```python
from build123d import *

# Parameters (mm, degrees)
SKETCH1_W           = 7.62
SKETCH1_H           = 19.05
BOSS_EXTRUDE1_DEPTH = 63.5
SKETCH2_R           = 0.889
CUT_EXTRUDE1_DEPTH  = 6.35
SKETCH3_R           = 3.3782
CUT_EXTRUDE2_DEPTH  = 8.62
SKETCH4_R           = 3.3782
CUT_EXTRUDE3_DEPTH  = 8.62


with BuildPart() as part:
    # Sketch1 → Boss-Extrude1 (new body)
    with BuildSketch(Plane.XY):
        with Locations((3.81, 9.525)):
            Rectangle(SKETCH1_W, SKETCH1_H)
    extrude(amount=-BOSS_EXTRUDE1_DEPTH)

    # Sketch2 → Cut-Extrude1 (cut)
    with BuildSketch(Plane.XY):
        with Locations((4.826, 11.43)):
            Circle(SKETCH2_R)
    extrude(amount=-CUT_EXTRUDE1_DEPTH, mode=Mode.SUBTRACT)

    # Sketch3 → Cut-Extrude2 (cut, through all)
    with BuildSketch(Plane.ZY):
        with Locations((-48.26, 12.7)):
            Circle(SKETCH3_R)
    extrude(amount=-CUT_EXTRUDE2_DEPTH, mode=Mode.SUBTRACT)

    # Sketch4 → Cut-Extrude3 (cut, through all)
    with BuildSketch(Plane.ZY):
        with Locations((-26.67, 12.7)):
            Circle(SKETCH4_R)
    extrude(amount=-CUT_EXTRUDE3_DEPTH, mode=Mode.SUBTRACT)


solid = part.part
```
Geometry: final body of the model. Coordinates: model frame, mm. A direction names the side the tool comes from. Round coordinates to 2 decimals unless told otherwise and drop trailing zeros. Order: outer loops, then holes, each group sorted by start corner. A loop starts at its lowest first (then second) coordinate and runs counter-clockwise, first axis right, second up. Notation, with made-up numbers: (10, -16.5) -> (68, -16.5) arc R33 cw to (68, 13.5) -> close; hole circle Ø6 at (70.5, 53). An arc over 180 degrees is marked (long way). Use one line per item in the form item = value. Start each with the question number.
1. Draft query along X for faces 1 (the face through (3.938, 11.469, -3.131)), 2 (the face through (0, 9, -31)), 3 (the face through (4, 0, -31)). Return one class per face: pulls with the +X half, pulls with the -X half, needs draft (parallel to the pull), parting line crosses it, or undercut.
2. Reachability of faces 4 (the face through (4, 19.05, -31)), 5 (the face through (5, 11, -6.35)) from +Z, -Z, +X, -X, +Y, -Y: full face, straight path, thin tool, end or side. Return the list, or none.
3. Line query: probe 1 along Z at (x, y) = (4.75, 14); probe 2 along Y at (x, z) = (2, -26.67); probe 3 along Z at (x, y) = (6.5, 13.25). Output: solid intervals per line, ascending.
4. Cut plane B-B (z = -26.67). Return the cut outline in (x, y), then the cut area to 3 significant figures.
5. Pin query (flat end, axial travel): pin 1 Ø9 at (y, z) = (12.7, -48.26) entering from -X; pin 2 Ø0.5 at (x, y) = (5, 12) entering from +Z. Return the tip coordinate at first contact, or that it passes through.
6. Cut plane C-C (y = 11.43). Return the cut outline in (x, z) (3 decimals).
7. Cut plane A-A (x = 2). Return the cut outline in (y, z), then the cut area to 3 significant figures.
Solution:
q1.face_1 = undercut
q1.face_2 = pulls with the -X half
q1.face_3 = needs draft
q2.face_4 = +Z, -Z, +X, -X, +Y
q2.face_5 = +Z
q3.probe_1 = -63.5 to -51.38, -45.14 to -29.79, -23.55 to 0
q3.probe_2 = 0 to 9.32, 16.08 to 19.05
q3.probe_3 = -63.5 to -51.59, -44.93 to -30, -23.34 to 0
q4.outline = (0, 0) -> (7.62, 0) -> (7.62, 9.32) -> (0, 9.32) -> close; (0, 16.08) -> (7.62, 16.08) -> (7.62, 19.05) -> (0, 19.05) -> close
q4.area = 93.7 mm^2
q5.pin_1 = 0
q5.pin_2 = -6.35
q6.outline = (0, -63.5) -> (7.62, -63.5) -> (7.62, -51.39) -> (0, -51.39) -> close; (0, -45.13) -> (7.62, -45.13) -> (7.62, -29.8) -> (0, -29.8) -> close; (0, -23.54) -> (7.62, -23.54) -> (7.62, 0) -> (5.715, 0) -> (5.715, -6.35) -> (3.937, -6.35) -> (3.937, 0) -> (0, 0) -> close
q7.outline = (0, -63.5) -> (19.05, -63.5) -> (19.05, 0) -> (0, 0) -> close; hole circle Ø6.76 at (12.7, -48.26); hole circle Ø6.76 at (12.7, -26.67)
q7.area = 1,140 mm^2
